The figure shows three views and two pictorial views of one solid part (mm, origin at its lowest corner). Answer the questions. A direction names the side the tool comes from. Coordinates: 2 decimals unless noted, no trailing zeros. Loops run counter-clockwise (first coordinate to the right, second up) from the corner with the lowest first, then second, coordinate; pieces in that order, holes last.
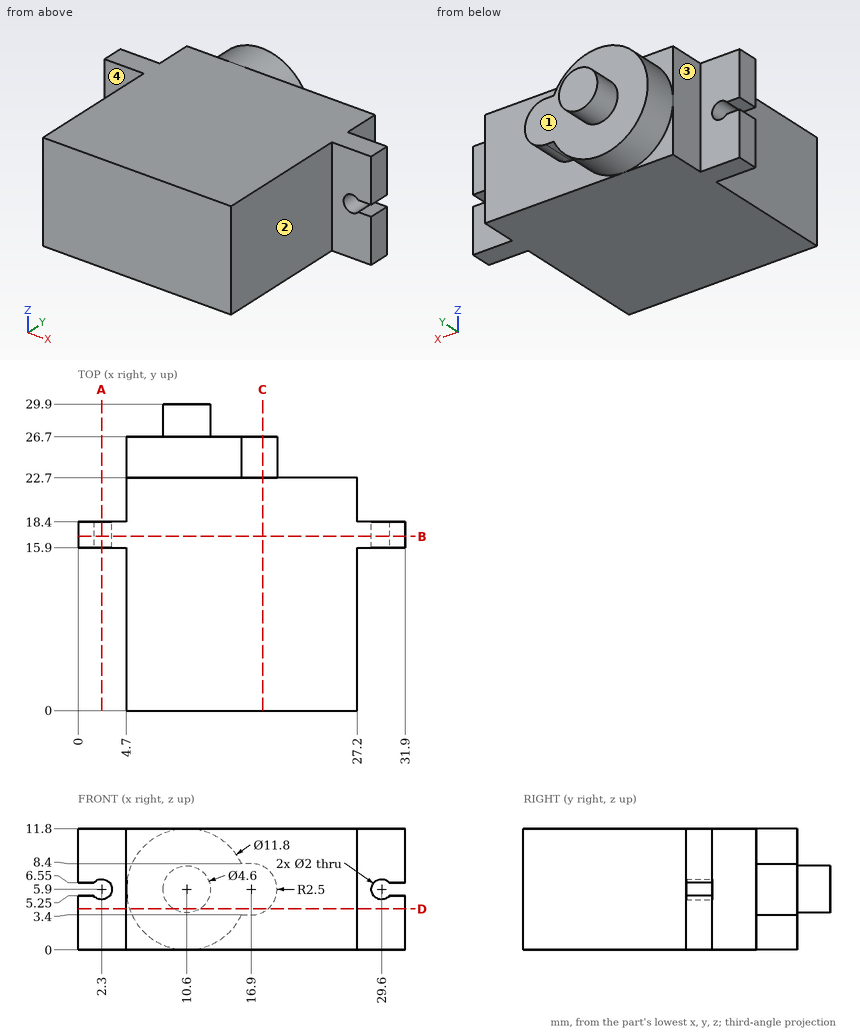
Q1. A cutting plane is placed at B-B (y = 17). Give the vertices of the cut face in (x, z), then the cut area to 3 significant figures.
Findings below:
outline: (0, 0) - (31.9, 0) - (31.9, 5.25) - (30.36, 5.25) arc R1 cw (long way) to (30.36, 6.55) - (31.9, 6.55) - (31.9, 11.8) - (0, 11.8) - (0, 6.55) - (1.54, 6.55) arc R1 cw (long way) to (1.54, 5.25) - (0, 5.25) - close
area: 367 mm2
Q2. Which of the six approach directions +Z, -Z, +X, -X, +Y, -Y give full straight-line access (tool end or side, diameter ignored) to the marked faces 1, 2, 3 and 4?
Findings below:
face 1: +Y
face 2: +Z, -Z, +X, -Y
face 3: +Z, -Z, -X, +Y
face 4: +Z, -Z, -X, -Y
Q3. Flat-ended cylindrical pins translate along their axes: pin 1 Ø0.8 at (x, y) = (16.5, 24.5) entering from -Z; pin 2 Ø2.5 at (x, z) = (30.5, 7.5) entering from -Y; pin 3 Ø3.5 at (y, z) = (21, 8.5) entering from -X. Find the tip coordinate at first contact, or state that the pin passes through.
Findings below:
pin 1: stops at z = 3.4
pin 2: stops at y = 15.9
pin 3: stops at x = 4.7
Q4. A cutting plane is placed at C-C (x = 18). Give the vertices of the cut face in (y, z) (3 decimals), then the cut area to 3 significant figures.
Findings below:
outline: (0, 0) - (22.7, 0) - (22.7, 3.655) - (26.7, 3.655) - (26.7, 8.145) - (22.7, 8.145) - (22.7, 11.8) - (0, 11.8) - close
area: 286 mm2
Q5. A cutting plane is placed at A-A (x = 2.3). Give the vertices of the cut face in (y, z).
Findings below:
outline: (15.9, 0) - (18.4, 0) - (18.4, 4.9) - (15.9, 4.9) - close; (15.9, 6.9) - (18.4, 6.9) - (18.4, 11.8) - (15.9, 11.8) - close
Q6. Straight lines are drawn through the part: probe 1 along Z at (x, y) = (2.3, 17.4); probe 2 along Y at (x, z) = (30, 1); probe 3 along X at (y, z) = (17.8, 5.9). For each, find the intervals that lie inside material, in ascending order.
Findings below:
probe 1: z = 0 to 4.9, 6.9 to 11.8
probe 2: y = 15.9 to 18.4
probe 3: x = 3.3 to 28.6
Q7. A cutting plane is placed at D-D (z = 4). Give the vertices of the cut face in (x, y), then the cut area to 3 significant figures.
Findings below:
outline: (0, 15.9) - (4.7, 15.9) - (4.7, 0) - (27.2, 0) - (27.2, 15.9) - (31.9, 15.9) - (31.9, 18.4) - (27.2, 18.4) - (27.2, 22.7) - (18.52, 22.7) - (18.52, 26.7) - (11.9, 26.7) - (11.9, 29.9) - (9.3, 29.9) - (9.3, 26.7) - (5.01, 26.7) - (5.01, 22.7) - (4.7, 22.7) - (4.7, 18.4) - (0, 18.4) - close
area: 597 mm2
